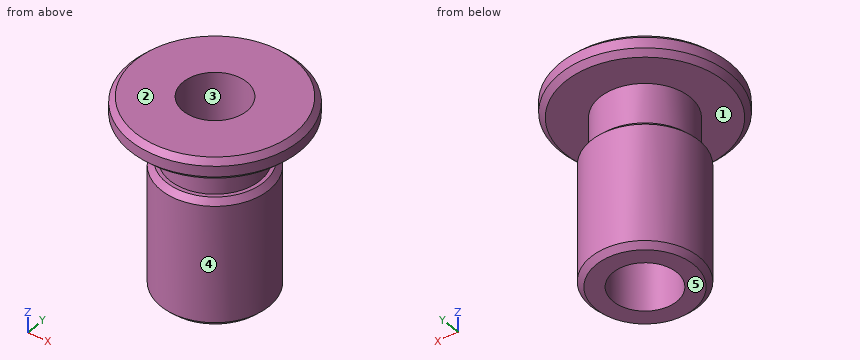
from build123d import *

# Parameters (mm, degrees)
F0_R     = 203.2
F1_DEPTH = 50.8
F2_R     = 107.95
F3_DEPTH = 101.6
F4_R     = 129.54
F5_DEPTH = 304.8
F6_R     = 76.2
F7_DEPTH = 457.2
F8_SIZE  = 12.7
F9_SIZE  = 12.7
F10_SIZE = 12.7


with BuildPart() as f1:
    # F0 (on Top) → F1 (new body)
    with BuildSketch(Plane.XY):
        Circle(F0_R)
    extrude(amount=F1_DEPTH)

    # F2 (on face) → F3 (join)
    with BuildSketch(Plane(origin=(0, 0, 0), x_dir=(1, 0, 0), z_dir=(0, 0, -1))):
        Circle(F2_R)
    extrude(amount=F3_DEPTH)

    # F4 (on face) → F5 (join)
    with BuildSketch(Plane(origin=(0, 0, -101.6), x_dir=(1, 0, 0), z_dir=(0, 0, -1))):
        Circle(F4_R)
    extrude(amount=F5_DEPTH)

    # F6 (on face) → F7 (cut)
    with BuildSketch(Plane.XY.offset(50.8)):
        Circle(F6_R)
    extrude(amount=-F7_DEPTH, mode=Mode.SUBTRACT)

    # F8
    f8_edges = [f1.edges().sort_by_distance(p)[0] for p in [
        (-203.2, 0, 50.8),
    ]]
    chamfer(f8_edges, length=F8_SIZE)

    # F9
    f9_edges = [f1.edges().sort_by_distance(p)[0] for p in [
        (-203.2, 0, 0),
    ]]
    chamfer(f9_edges, length=F9_SIZE)

    # F10
    f10_edges = [f1.edges().sort_by_distance(p)[0] for p in [
        (-129.54, 0, -101.6),
        (-129.54, 0, -406.4),
    ]]
    chamfer(f10_edges, length=F10_SIZE)


solid = f1.part
Geometry: final body of the model. Coordinates: model frame, mm. Face numbers are marked on the shaded views. A direction names the side the tool comes from. Coordinates: 2 decimals unless noted, no trailing zeros. Write each loop counter-clockwise with the first axis right and the second up, starting at its lowest first coordinate (ties: lowest second). Pieces come first, ordered by that corner, then holes. Notation, with made-up numbers: (-19, 21.5) - (18, 21.5) arc R17 cw to (18, 43.5) - close; hole circle Ø5 at (-12.75, 80). An arc over 180 degrees is marked (long way). Return JSON: item names as keys, results as strings.
Item 1: Line query: L1, parallel to Y at x = 0, z = -152; L2, parallel to Y at x = 0, z = -51; L3, parallel to Z at x = 100.5, y = 104.5. Output: solid intervals per line, ascending.
Completed:
{"L1": "y = -129.54 to -76.2, 76.2 to 129.54", "L2": "y = -107.95 to -76.2, 76.2 to 107.95", "L3": "z = 0 to 50.8"}
Item 2: Section query C-C (z = -168). Output: boundary loops of the cut face in (x, y), and give its area (3 significant figures).
Completed:
{"outline": "circle Ø259.08 at (0, 0); hole circle Ø152.4 at (0, 0)", "area": "34,500 mm2"}
Item 3: Reachability of the marked faces 1 and 2 from +Z, -Z, +X, -X, +Y, -Y: full face, straight path, thin tool, end or side. Return the list, or none.
Completed:
{"face 1": "none", "face 2": "+Z, +X, -X, +Y, -Y"}
Item 4: Section query A-A (x = 0). Output: boundary loops of the cut face in (y, z).
Completed:
{"outline": "(-203.2, 12.7) - (-190.5, 0) - (-107.95, 0) - (-107.95, -101.6) - (-116.84, -101.6) - (-129.54, -114.3) - (-129.54, -393.7) - (-116.84, -406.4) - (-76.2, -406.4) - (-76.2, 50.8) - (-190.5, 50.8) - (-203.2, 38.1) - close; (76.2, -406.4) - (116.84, -406.4) - (129.54, -393.7) - (129.54, -114.3) - (116.84, -101.6) - (107.95, -101.6) - (107.95, 0) - (190.5, 0) - (203.2, 12.7) - (203.2, 38.1) - (190.5, 50.8) - (76.2, 50.8) - close"}
Item 5: Pull-direction query (X, two-part tool) for the marked faces 3, 4 and 5; classes: +X half, -X half, draft (parallel to the pull), parting line (faces both ways), or undercut.
Completed:
{"face 3": "undercut", "face 4": "parting line", "face 5": "draft"}
Item 6: Pin query (flat end, axial travel): pin 1 Ø5 at (y, z) = (-44.5, -233.5) entering from -X; pin 2 Ø2 at (y, z) = (84, -93.5) entering from -X; pin 3 Ø5 at (y, z) = (86, -14.5) entering from +X. Return the tip coordinate at first contact, or that it passes through.
Completed:
{"pin 1": "stops at x = -122.54", "pin 2": "stops at x = -69.02", "pin 3": "stops at x = 68.42"}
Item 7: Section query D-D (z = -44). Output: boundary loops of the cut face in (x, y).
Completed:
{"outline": "circle Ø215.9 at (0, 0); hole circle Ø152.4 at (0, 0)"}
